```python
from build123d import *

# Parameters (mm, degrees)
BOSS_EXTRU_1_DEPTH         = 67
ENL_V_MAT_EXTRU_1_REACH    = 111.037
ESQUISSE2_R                = 3.15
ENL_V_MAT_EXTRU_3_DEPTH    = 1.5
ESQUISSE12_W               = 4.842495097
ESQUISSE12_H               = 1.5
R_P_TITION_LIN_AIRE1_COUNT = 2
R_P_TITION_LIN_AIRE1_PITCH = 42


with BuildPart() as part:
    # Esquisse1 → Boss.-Extru.1 (new body)
    with BuildSketch(Plane.XY):
        with BuildLine():
            Line((0, 0), (50, 0))
            Line((50, 0), (50, 17.5))
            Line((50, 17.5), (43.454482672, 17.5))
            ThreePointArc((43.454482672, 17.5), (8, 27), (43.454482672, 36.5))
            Line((43.454482672, 36.5), (50, 36.5))
            Line((50, 36.5), (50, 54.2))
            Line((50, 54.2), (21, 54.2))
            Line((21, 54.2), (21, 57.5))
            Line((21, 57.5), (50, 57.5))
            Line((50, 57.5), (50, 70))
            Line((50, 70), (0, 70))
            Line((0, 70), (0, 0))
        make_face()
    extrude(amount=BOSS_EXTRU_1_DEPTH)

    # Esquisse2 → Enlèv. mat.-Extru.1 (cut, up to next)
    with BuildSketch(Plane(origin=(0, 70, 0), x_dir=(1, 0, 0), z_dir=(0, 1, 0)), mode=Mode.PRIVATE) as enl_v_mat_extru_1_sk1:
        with Locations(Location((41.7, -33.5, 0), (0, 0, 270))):
            Circle(ESQUISSE2_R)
    enl_v_mat_extru_1_tool1 = extrude(enl_v_mat_extru_1_sk1.sketch, amount=-ENL_V_MAT_EXTRU_1_REACH, mode=Mode.PRIVATE) & part.part
    add(enl_v_mat_extru_1_tool1.solids().sort_by_distance((41.7, 70, 33.5))[0], mode=Mode.SUBTRACT)

    # Esquisse8 → Enlèv. mat.-Extru.3 (cut)
    with BuildSketch(Plane.ZY):
        Polygon((63.532395101, 73.318993261), (33.5, 41.941864051), (3.467604899, 73.318993261), (-3.467604899, 66.681006739), (26.855644409, 35), (-3.467604899, 3.318993261), (3.467604899, -3.318993261), (33.5, 28.058135949), (63.532395101, -3.318993261), (70.467604899, 3.318993261), (40.144355591, 35), (70.467604899, 66.681006739), align=None)
    extrude(amount=-ENL_V_MAT_EXTRU_3_DEPTH, mode=Mode.SUBTRACT)

    # Esquisse12 → Enlèvement de matière-Révolution2 (revolve, cut)
    with BuildSketch(Plane(origin=(0, 27, 0), x_dir=(1, 0, 0), z_dir=(0, 1, 0))):
        with Locations((44.070102797, -53.75)):
            Rectangle(ESQUISSE12_W, ESQUISSE12_H)
    enl_vement_de_mati_re_r_volution2 = revolve(axis=Axis((26.491350346, 27, 66.236309337), (0, 0, -1)), mode=Mode.SUBTRACT)

    # Répétition linéaire1: Enlèvement de matière-Révolution2 ×2
    with Locations(*[(0, 0, -i * R_P_TITION_LIN_AIRE1_PITCH) for i in range(1, R_P_TITION_LIN_AIRE1_COUNT)]):
        add(enl_vement_de_mati_re_r_volution2, mode=Mode.SUBTRACT)


solid = part.part
```
CAD build for the part. Positions are in the model's coordinates, mm. A direction names the side the tool comes from. Coordinates: 2 decimals unless noted, no trailing zeros. Order: outer loops, then holes, each group sorted by start corner. A loop starts at its lowest first (then second) coordinate and runs counter-clockwise, first axis right, second up. Notation, with made-up numbers: (-18.75, 34) -> (4.25, 34) arc R10 ccw to (4.25, 50) -> close; hole circle Ø1 at (61.25, -33). An arc over 180 degrees is marked (long way). Use one line per item in the form item = value. Start each with the question number.
1) Band-saw the part on D-D on y = 56.5. Give the cut face in (x, z).
2) Pull direction X, two halves, no side cores. Call faces 1 (the flat face through (50, 64, 33)), 2 (the cylindrical face through (6.505, 26.259, 11.74)), 3 (the flat face through (0.74, 20.775, 53.76)), 4 (the flat face through (0, 35, 10)): +X half, -X half, draft (parallel to the pull), parting line (faces both ways), or undercut.
3) Drop flat-ended pins along their axis: pin 1 (3.5 mm diameter, centred on y = 55.5, z = 48.5, fed in from +X); pin 2 (5 mm diameter, centred on y = 30, z = 54, fed in from +X); pin 3 (5.5 mm diameter, centred on x = 41.7, z = 33.5, fed in from +Y). Give the stop position or say it passes through.
4) Tool access for faces 5 (the flat face through (8.7, 32.8, 11)), 6 (the flat face through (0.74, 56.17, 47.12)), 7 (the flat face through (21, 56, 33)), 8 (the cylindrical face through (8.013, 26.304, 5.423)): list every direction of +Z, -Z, +X, -X, +Y, -Y with a clear straight run to the whole face (end or side of a thin tool).
5) Drill centre lines: L1, parallel to Y at x = 46, z = 23; L2, parallel to Y at x = 29, z = 29.5; L3, parallel to X at y = 4, z = 5. Where is each one in solid material? Low to high. Write a range as [from, to].
6) Band-saw the part on A-A on x = 41.7. State how many separate pieces and enclosed holes the cut face has, then the cut area to 3 significant figures.
7) Band-saw the part on B-B on y = 40.5. Give the cut face in (x, z) (3 decimals).
8) Band-saw the part on C-C on x = 14.5. Give the cut face in (y, z).
Entries:
q1.outline = (0, 0) -> (21, 0) -> (21, 67) -> (0, 67) -> (0, 60.72) -> (1.5, 60.72) -> (1.5, 47.43) -> (0, 47.43) -> (0, 19.57) -> (1.5, 19.57) -> (1.5, 6.28) -> (0, 6.28) -> close
q2.face_1 = +X half
q2.face_2 = undercut
q2.face_3 = draft
q2.face_4 = -X half
q3.pin_1 = 50
q3.pin_2 = 8.8
q3.pin_3 = 54.2
q4.face_5 = none
q4.face_6 = -X
q4.face_7 = +Z, -Z, +X
q4.face_8 = +Z, -Z
q5.L1 = [0, 17.5], [36.5, 54.2], [57.5, 70]
q5.L2 = [0, 8.11], [45.89, 54.2], [57.5, 70]
q5.L3 = [1.5, 50]
q6.separate_pieces = 4
q6.enclosed_holes = 0
q6.area = 2,770 mm2
q7.outline = (0, 0) -> (13.63, 0) -> (13.63, 11) -> (11.735, 11) -> (11.735, 12.5) -> (13.63, 12.5) -> (13.63, 53) -> (11.735, 53) -> (11.735, 54.5) -> (13.63, 54.5) -> (13.63, 67) -> (0, 67) -> (0, 45.409) -> (1.5, 45.409) -> (1.5, 21.591) -> (0, 21.591) -> close; (40.37, 0) -> (50, 0) -> (50, 67) -> (40.37, 67) -> (40.37, 54.5) -> (41.248, 54.5) -> (41.248, 53) -> (40.37, 53) -> (40.37, 12.5) -> (41.248, 12.5) -> (41.248, 11) -> (40.37, 11) -> close
q8.outline = (0, 0) -> (12.69, 0) -> (12.69, 11) -> (10.99, 11) -> (10.99, 12.5) -> (12.69, 12.5) -> (12.69, 53) -> (10.99, 53) -> (10.99, 54.5) -> (12.69, 54.5) -> (12.69, 67) -> (0, 67) -> close; (41.31, 0) -> (70, 0) -> (70, 67) -> (41.31, 67) -> (41.31, 54.5) -> (43.01, 54.5) -> (43.01, 53) -> (41.31, 53) -> (41.31, 12.5) -> (43.01, 12.5) -> (43.01, 11) -> (41.31, 11) -> close
